The drawing under review shows one solid part. Ordinate dimensions are in mm from its lowest x, y, z. Round coordinates to 2 decimals unless told otherwise and drop trailing zeros. Write each loop counter-clockwise with the first axis right and the second up, starting at its lowest first coordinate (ties: lowest second). Pieces come first, ordered by that corner, then holes. Notation, with made-up numbers: (-22.5, 53.5) - (21.5, 53.5) arc R17 ccw to (21.5, 75.5) - close; hole circle Ø6 at (-9.5, -35). An arc over 180 degrees is marked (long way). One line per question, with ' | ' between items. Start each with the question number.
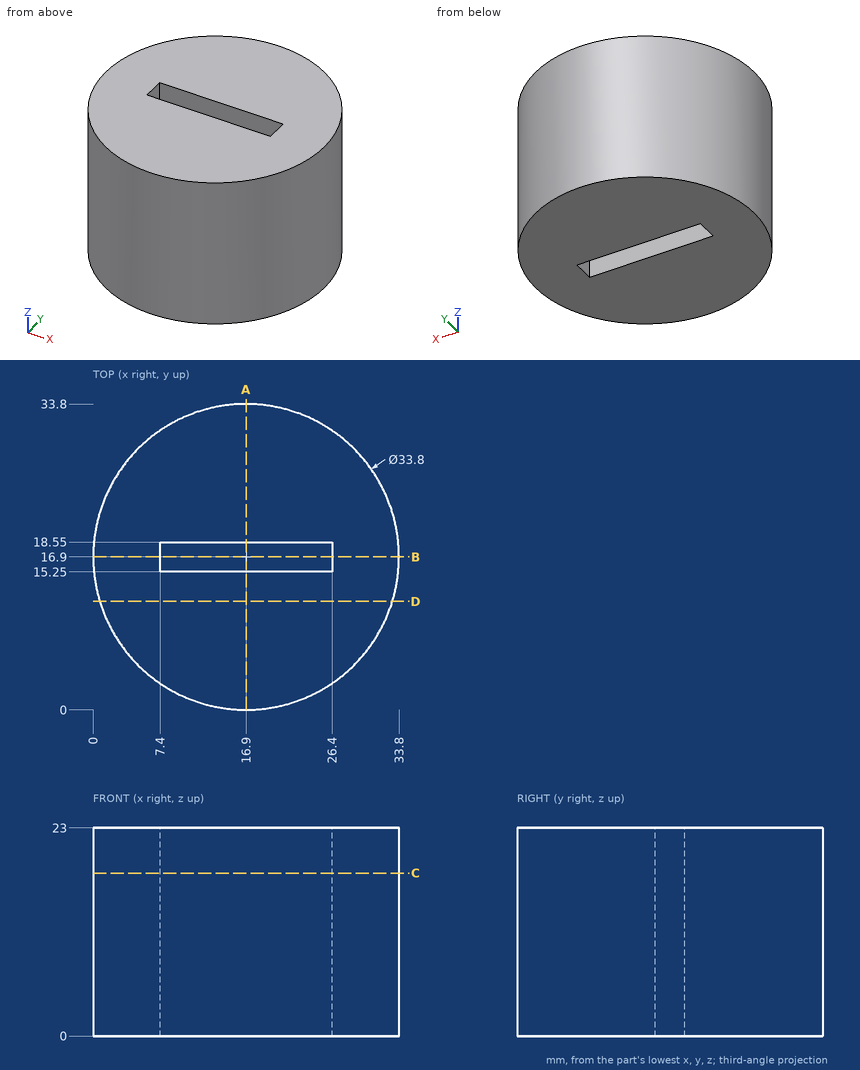
1. Clearance check with flat-ended pins moving along their axes: P1, Ø1.5, axis at x = 15, y = 22.5, coming from the -Z side; P2, Ø4, axis at x = 5.5, z = 18.5, coming from the +Y side; P3, Ø4, axis at y = 10, z = 11, coming from the +X side; P4, Ø1.5, axis at y = 15, z = 16.5, coming from the -X side. State where each tip first meets the part, or that it passes through.
2. Add section A-A, the plane x = 16.9. Write out the cut boundary in (y, z), then the cut area to 4 significant figures.
3. Add section D-D, the plane y = 12. Write out the cut boundary in (x, z), then the cut area to 3 significant figures.
4. Add section B-B, the plane y = 16.9. Write out the cut boundary in (x, z), then the cut area to 3 significant figures.
5. Wall thickness on line 1 along Y through (x, z) = (17, 6.25); line 2 along Y through (x, z) = (9.5, 16.25); line 3 along X through (y, z) = (23, 4.75): over which ranges is each line inside the solid? List them lowest first. Write a range as [from, to].
6. Add section C-C, the plane z = 18. Write out the cut boundary in (x, y).
Geometry check:
1) P1: stops at z = 0 | P2: stops at y = 30.94 | P3: stops at x = 33.07 | P4: stops at x = 0.04
2) outline: (0, 0) - (15.25, 0) - (15.25, 23) - (0, 23) - close; (18.55, 0) - (33.8, 0) - (33.8, 23) - (18.55, 23) - close | area: 701.5 mm2
3) outline: (0.73, 0) - (33.07, 0) - (33.07, 23) - (0.73, 23) - close | area: 744 mm2
4) outline: (0, 0) - (7.4, 0) - (7.4, 23) - (0, 23) - close; (26.4, 0) - (33.8, 0) - (33.8, 23) - (26.4, 23) - close | area: 340 mm2
5) line 1: y = [0, 15.25], [18.55, 33.8] | line 2: y = [1.71, 15.25], [18.55, 32.09] | line 3: x = [1.14, 32.66]
6) outline: circle Ø33.8 at (16.9, 16.9); hole (7.4, 15.25) - (26.4, 15.25) - (26.4, 18.55) - (7.4, 18.55) - close
